from build123d import *

# Parameters (mm, degrees)
SKETCH_2_R          = 1.5
CUT_EXTRUDE_1_DEPTH = 5


with BuildPart() as part:
    # Эскиз1 → Повернуть1 (revolve)
    with BuildSketch(Plane(origin=(0, 0, 0), x_dir=(0, 0, -1), z_dir=(1, 0, 0))):
        Polygon((0.7, 13), (0, 13), (0, 7), (0.7, 7), (0.7, 0), (1, 0), (1, 23), (0.7, 23), align=None)
    revolve(axis=Axis((0, 0, 0), (0, 1, 0)))

    # Эскиз2 → Вырез-Вытянуть1 (cut, symmetric)
    with BuildSketch(Plane.XY):
        with Locations((1.5, 3)):
            Circle(SKETCH_2_R)
    extrude(amount=CUT_EXTRUDE_1_DEPTH, both=True, mode=Mode.SUBTRACT)


solid = part.part
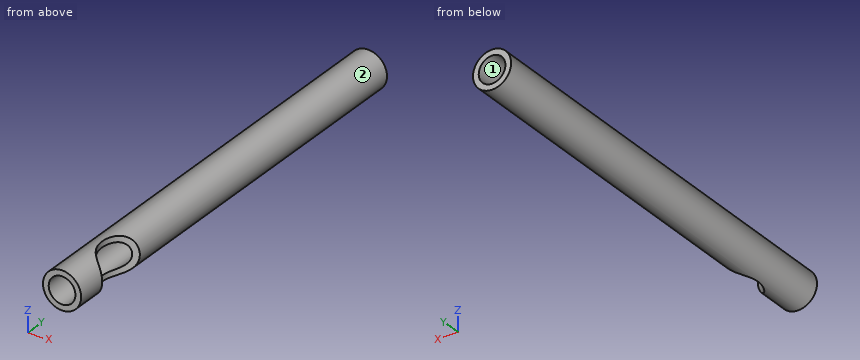
Geometry: final body of the model. Coordinates: model frame, mm. Face numbers are marked on the shaded views. Give positions to 0.01 mm unless a question says otherwise; leave off trailing zeros. Loops run counter-clockwise (first coordinate to the right, second up) from the corner with the lowest first, then second, coordinate; pieces in that order, holes last. Notation, with made-up numbers: (-35.5, -21) - (16.5, -21) arc R27 ccw to (16.5, 8) - close; hole circle Ø1 at (85.25, -39.75). An arc over 180 degrees is marked (long way). Answer as CSV lines item,"result". Start each with the question number.
1. Ray query, L1, parallel to X at y = 19.75, z = 0; L2, parallel to Y at x = -0.1, z = 0.15. Return the intervals inside material, ascending.
2. Section A-A, the plane x = 0.35. Return loops of the section in (y, z).
3. Section B-B, the plane z = -0.15. Return loops of the section in (x, y).
4. Section C-C, the plane y = 14.5. Return loops of the section in (x, z), plus the area to 3 significant figures.
5. Draft query along X for the marked faces 1 and 2. Return one class per face: released by +X, released by -X, zero draft, split by the parting line, or undercut.
6. Pin query (flat end, axial travel): P1, Ø1.1, axis at x = 0, z = 0, coming from the +Y side. Return the tip coordinate at first contact, or that it passes through.
Answers:
1,L1,"x = -1 to -0.7, 0.7 to 1"
1,L2,"y = 7 to 13"
2,outline,"(0, -0.94) - (2.04, -0.94) - (2.04, -0.61) - (0, -0.61) - close; (0, 0.61) - (2.04, 0.61) - (2.04, 0.94) - (0, 0.94) - close; (3.96, -0.94) - (23, -0.94) - (23, -0.61) - (13, -0.61) - (13, 0.61) - (23, 0.61) - (23, 0.94) - (3.96, 0.94) - (3.96, 0.61) - (7, 0.61) - (7, -0.61) - (3.96, -0.61) - close"
3,outline,"(-0.99, 0) - (-0.68, 0) - (-0.68, 7) - (0.68, 7) - (0.68, 4.26) arc R1.5 cw to (0.99, 4.41) - (0.99, 23) - (0.68, 23) - (0.68, 13) - (-0.68, 13) - (-0.68, 23) - (-0.99, 23) - close; (0.68, 0) - (0.99, 0) - (0.99, 1.59) arc R1.5 cw to (0.68, 1.74) - close"
4,outline,"circle Ø2 at (0, 0); hole circle Ø1.4 at (0, 0)"
4,area,"1.60 mm2"
5,face 1,"undercut"
5,face 2,"split by the parting line"
6,P1,"stops at y = 13"
